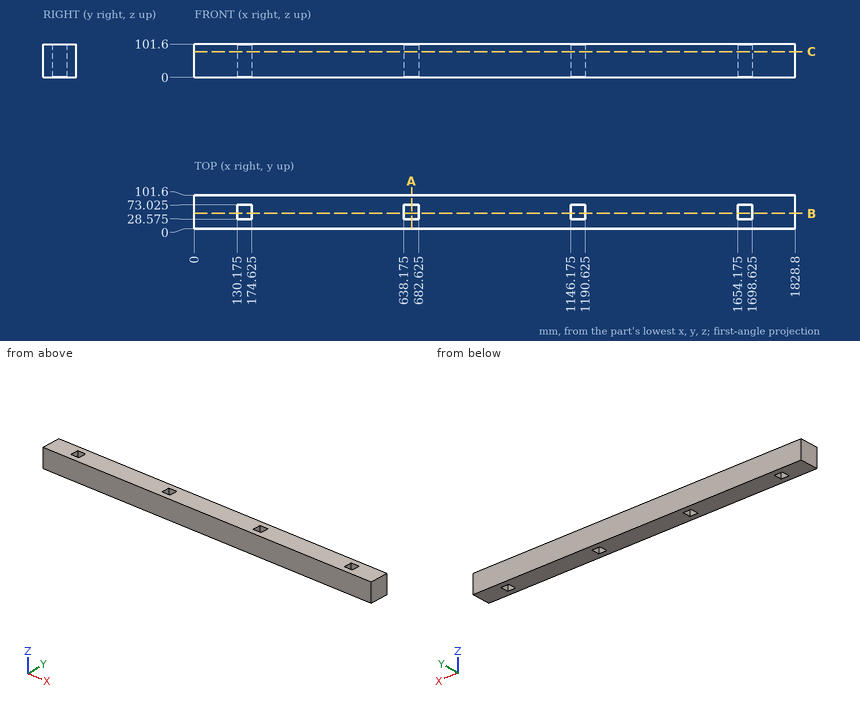
Geometry check sheet. Reference: drawing and pictorial views, mm from the part's lowest x, y, z. Give positions to 0.01 mm unless a question says otherwise; leave off trailing zeros. Order: outer loops, then holes, each group sorted by start corner. A loop starts at its lowest first (then second) coordinate and runs counter-clockwise, first axis right, second up. Notation, with made-up numbers: M -32.5,49 L 19.5,49 A18 cw 19.5,67 Z; hole C -4,60.5 d2. An arc over 180 degrees is marked long. Answer in a Markdown table with one row per item. Add a question column.
Item 1: Gauge pin test, flat end, axial feed: pin 1 (13.5 mm diameter, centred on x = 1669.5, z = 51.5, fed in from -Y). Record the tip position at first contact, or that the pin passes through.
Item 2: Section check A-A, the plane x = 661.5. Enter the section's corners in (y, z) (3 decimals).
Item 3: Section check B-B, the plane y = 47. Enter the section's corners in (x, z) (3 decimals), and give its area (3 significant figures).
Item 4: Scan line: probe 1 along X at (y, z) = (56, 79.5) (3 decimals). Record every from-to range of solid material in increasing order. Write a range as from..to.
Item 5: Section check C-C, the plane z = 78.5. Enter the section's corners in (x, y) (3 decimals), and give its area (3 significant figures).
Filled sheet:
| question | item | result |
|---|---|---|
| 1 | pin 1 | stops at y = 0 |
| 2 | outline | M 0,0 L 28.575,0 L 28.575,101.6 L 0,101.6 Z; M 73.025,0 L 101.6,0 L 101.6,101.6 L 73.025,101.6 Z |
| 3 | outline | M 0,0 L 130.175,0 L 130.175,101.6 L 0,101.6 Z; M 174.625,0 L 638.175,0 L 638.175,101.6 L 174.625,101.6 Z; M 682.625,0 L 1146.175,0 L 1146.175,101.6 L 682.625,101.6 Z; M 1190.625,0 L 1654.175,0 L 1654.175,101.6 L 1190.625,101.6 Z; M 1698.625,0 L 1828.8,0 L 1828.8,101.6 L 1698.625,101.6 Z |
| 3 | area | 168,000 mm^2 |
| 4 | probe 1 | x = 0..130.175, 174.625..638.175, 682.625..1146.175, 1190.625..1654.175, 1698.625..1828.8 |
| 5 | outline | M 0,0 L 1828.8,0 L 1828.8,101.6 L 0,101.6 Z; hole M 130.175,28.575 L 174.625,28.575 L 174.625,73.025 L 130.175,73.025 Z; hole M 638.175,28.575 L 682.625,28.575 L 682.625,73.025 L 638.175,73.025 Z; hole M 1146.175,28.575 L 1190.625,28.575 L 1190.625,73.025 L 1146.175,73.025 Z; hole M 1654.175,28.575 L 1698.625,28.575 L 1698.625,73.025 L 1654.175,73.025 Z |
| 5 | area | 178,000 mm^2 |
